from build123d import *

# Parameters (mm, degrees)
BOSS_EXTRUDE1_DEPTH = 20
FILLET1_R           = 1


with BuildPart() as part:
    # Sketch1 → Boss-Extrude1 (new body)
    with BuildSketch(Plane.XY):
        with BuildLine():
            ThreePointArc((0, 10.635), (-10, 0.635), (0, -9.365))
            ThreePointArc((0, -9.365), (27.5, -36.865), (0, -64.365))
            ThreePointArc((0, -64.365), (-10, -74.365), (0, -84.365))
            ThreePointArc((0, -84.365), (47.5, -36.865), (0, 10.635))
        make_face()
        with BuildLine():
            ThreePointArc((1.072380529, 1.535), (0, -0.765), (-1.072380529, 1.535))
            Line((-1.072380529, 1.535), (1.072380529, 1.535))
        make_face(mode=Mode.SUBTRACT)
    extrude(amount=BOSS_EXTRUDE1_DEPTH)

    # Fillet1
    fillet1_edges = [part.edges().sort_by_distance(p)[0] for p in [
        (-10, 0.635, 20),
        (27.5, -36.865, 20),
        (-10, -74.365, 20),
        (47.5, -36.865, 20),
        (47.5, -36.865, 0),
        (-10, -74.365, 0),
        (27.5, -36.865, 0),
        (-10, 0.635, 0),
    ]]
    fillet(fillet1_edges, radius=FILLET1_R)


solid = part.part
Geometry check sheet. Reference: the model listing, model coordinates, mm. A direction names the side the tool comes from. Give positions to 0.01 mm unless a question says otherwise; leave off trailing zeros. Order: outer loops, then holes, each group sorted by start corner. A loop starts at its lowest first (then second) coordinate and runs counter-clockwise, first axis right, second up. Notation, with made-up numbers: (77.5, 17.25) - (89.5, 17.25) arc R26 cw to (89.5, 40.25) - close; hole circle Ø5 at (78, 60.5). An arc over 180 degrees is marked (long way). Use one line per item in the form item = value.
1) Depth check by flat-ended pin: pin 1 Ø10 at (x, z) = (6.5, 17) entering from -Y; pin 2 Ø3 at (x, z) = (40, 13.5) entering from +Y; pin 3 Ø2 at (y, z) = (-7.5, 13.5) entering from +X. Enter the tip coordinate at first touch or a pass-through.
Working result:
pin_1 = -84.34
pin_2 = -9.04
pin_3 = 38.1
2) Draft check along Y on faces 3 (the face through (47.49, -37.91, 9.87)), 4 (the face through (31, -36, 0)), 5 (the face through (0.044, -0.764, 9.86)). Enter one of: released by +Y, released by -Y, zero draft, split by the parting line, or undercut.
Working result:
face_3 = split by the parting line
face_4 = zero draft
face_5 = undercut
3) Material ranges on probe 1 along Y at (x, z) = (-1, 19.25) (3 decimals); probe 2 along Y at (x, z) = (6, 9); probe 3 along Y at (x, z) = (0.5, 2) (3 decimals), recorded low to high. Write a range as from..to.
Working result:
probe_1 = -84.283..-64.447, -9.283..-0.345, 1.535..10.553
probe_2 = -83.98..-63.7, -10.03..10.25
probe_3 = -84.362..-64.36, -9.37..-0.673, 1.535..10.632
4) Sectioned sample at A-A (z = 15.5). Record the boundary of the cut face in (x, y) (3 decimals).
Working result:
outline = (0, -84.365) arc R47.5 ccw to (0, 10.635) arc R10 ccw to (0, -9.365) arc R27.5 cw to (0, -64.365) arc R10 ccw to start; hole (-1.072, 1.535) arc R1.4 ccw (long way) to (1.072, 1.535) - close
5) Access from +Z, -Z, +X, -X, +Y, -Y to the whole of each face (thin tool, end or side, straight path). Record for faces 1 (the face through (-9.998, 0.855, 9.874)), 2 (the face through (0, 1.535, 10)).
Working result:
face_1 = +Z, -Z, -X
face_2 = +Z, -Z
